The listing builds one solid part. Answer for the finished solid, in the listing's coordinates (mm). A direction names the side the tool comes from. Round coordinates to 2 decimals unless told otherwise and drop trailing zeros. Order: outer loops, then holes, each group sorted by start corner. A loop starts at its lowest first (then second) coordinate and runs counter-clockwise, first axis right, second up. Notation, with made-up numbers: (-39, 77) - (-18, 77) arc R15 ccw to (-18, 100) - close; hole circle Ø4 at (35.5, 68). An arc over 180 degrees is marked (long way). Use CSV: the item, a comma, the result in double quotes. Start each with the question number.
Item 1: Find section C-C, the plane z = 35.5. Give the vertices of the cut face in (x, y), plus the area to 3 significant figures.
Item 2: For faces 1 (the flat face through (48.042, 4, 13)), 2 (the cylindrical face through (-16.68, 0.73, 39.4)), determine the directions among +Z, -Z, +X, -X, +Y, -Y from which every point of the face is accessible in a straight line to the end or side of a thin tool.
Item 3: Find section D-D, the plane y = -26. Give the vertices of the cut face in (x, z), plus the area to 3 significant figures.
Item 4: Find section B-B, the plane x = 0. Give the vertices of the cut face in (y, z), plus the area to 3 significant figures.
Item 5: Flat-ended cylindrical pins translate along their axes: P1, Ø8, axis at y = 8.5, z = 38, coming from the +X side; P2, Ø4, axis at x = -9.5, z = 54, coming from the +Y side; P3, Ø1.5, axis at y = -8, z = 27.5, coming from the -X side. Find the tip coordinate at first contact, or state that the pin passes through.
Item 6: Straight lines are drawn through the part: line 1 along Z through (x, y) = (-33.5, -11.5); line 2 along X through (y, z) = (-1, 49); line 3 along X through (y, z) = (3, 36). For each, find the intervals that lie inside material, in ascending order. Write a range as [from, to].
Item 7: Find section A-A, the plane y = 14. Give the vertices of the cut face in (x, z), plus the area to 3 significant figures.
```python
from build123d import *

# Parameters (mm, degrees)
F0_W     = 96.682288
F0_H     = 76.328121
F1_DEPTH = 25.4
F2_R     = 16.695936
F3_DEPTH = 38.1
F5_DEPTH = 38.1


with BuildPart() as f1:
    # F0 (on Top) → F1 (new body)
    with BuildSketch(Plane.XY):
        with Locations((-0.299327, 4.340227)):
            Rectangle(F0_W, F0_H)
    extrude(amount=F1_DEPTH)

    # F2 (on face) → F3 (join)
    with BuildSketch(Plane.XY.offset(25.4)):
        Circle(F2_R)
    extrude(amount=F3_DEPTH)

    # F4 (on Front) → F5 (cut, symmetric)
    with BuildSketch(Plane.XZ):
        Polygon((41.456647, 69.144301), (-32.776196, 69.144301), (41.456647, 35.021137), align=None)
    extrude(amount=F5_DEPTH, both=True, mode=Mode.SUBTRACT)


solid = f1.part
```
Worked out:
1,outline,"circle Ø33.39 at (0, 0)"
1,area,"876 mm²"
2,face 1,"+Z, -Z, +X, +Y, -Y"
2,face 2,"+Z"
3,outline,"(-48.64, 0) - (48.04, 0) - (48.04, 25.4) - (-48.64, 25.4) - close"
3,area,"2,460 mm²"
4,outline,"(-33.82, 0) - (42.5, 0) - (42.5, 25.4) - (16.7, 25.4) - (16.7, 54.08) - (-16.7, 54.08) - (-16.7, 25.4) - (-33.82, 25.4) - close"
4,area,"2,900 mm²"
5,P1,"stops at x = 16.08"
5,P2,"stops at y = 14.92"
5,P3,"stops at x = -15.04"
6,line 1,"z = [0, 25.4]"
6,line 2,"x = [-16.67, 11.05]"
6,line 3,"x = [-16.42, 16.42]"
7,outline,"(-48.64, 0) - (48.04, 0) - (48.04, 25.4) - (9.1, 25.4) - (9.1, 49.9) - (-9.1, 58.26) - (-9.1, 25.4) - (-48.64, 25.4) - close"
7,area,"2,980 mm²"
